Work out the finished part from the listing and answer in its coordinate system (mm). A direction names the side the tool comes from. Coordinates: 2 decimals unless noted, no trailing zeros. Write each loop counter-clockwise with the first axis right and the second up, starting at its lowest first coordinate (ties: lowest second). Pieces come first, ordered by that corner, then holes. Notation, with made-up numbers: M 14.25,-25 L 61.25,-25 A12 cw 61.25,-6 Z; hole C 35,50.25 d2. An arc over 180 degrees is marked long. Use CSV: the item, a comma, the result in double quotes.
from build123d import *

# Parameters (mm, degrees)
F0_R     = 11
F1_DEPTH = 5
F3_DEPTH = 3.5
F5_DEPTH = 14.501
F6_R     = 2.5
F7_DEPTH = 14.501
F8_R     = 8
F9_DEPTH = 25
F10_SIZE = 2


with BuildPart() as f1:
    # F0 (on Top) → F1 (new body)
    with BuildSketch(Plane.XY):
        Circle(F0_R)
    extrude(amount=F1_DEPTH)

    # F2 (on Right) → F3 (join, symmetric)
    with BuildSketch(Plane.YZ):
        Polygon((-11, 5), (0, 5), (11, 5), (11, 40), (-11, 40), align=None)
    extrude(amount=F3_DEPTH, both=True)

    # F4 (on face) → F5 (cut, through all)
    with BuildSketch(Plane.YZ.offset(3.5)):
        Polygon((-11, 35), (0, 40), (-11, 40), align=None)
    extrude(amount=-F5_DEPTH, mode=Mode.SUBTRACT)

    # F6 (on face) → F7 (cut, through all)
    with BuildSketch(Plane.YZ.offset(3.5)):
        with Locations((0, 20)):
            Circle(F6_R)
    extrude(amount=-F7_DEPTH, mode=Mode.SUBTRACT)

    # F8 (on face) → F9 (join)
    with BuildSketch(Plane(origin=(0, 0, 0), x_dir=(1, 0, 0), z_dir=(0, 0, -1))):
        Circle(F8_R)
    extrude(amount=F9_DEPTH)

    # F10
    f10_edges = [f1.edges().sort_by_distance(p)[0] for p in [
        (-8, 0, -25),
    ]]
    chamfer(f10_edges, length=F10_SIZE)


solid = f1.part
Item 1: Consider probe 1 along Z at (x, y) = (1.5, 0); probe 2 along X at (y, z) = (-6.75, 34); probe 3 along Z at (x, y) = (9.5, 5.25). Determine where each line is inside the solid, lowest interval first.
Answer:
probe 1,"z = -25 to 17.5, 22.5 to 40"
probe 2,"x = -3.5 to 3.5"
probe 3,"z = 0 to 5"
Item 2: A tool of negligible diameter and unlimited length cuts with its end or side. For faces 4 (the face through (3.5, 0, 23)), 5 (the face through (-6, 0, 5)), 6 (the face through (-2, -8, 0)), 7 (the face through (0.049, -5.577, 37.465)), from which of +Z, -Z, +X, -X, +Y, -Y can it reach the whole face along a straight path? Write none if from no direction.
Answer:
face 4,"+Z, +X, +Y, -Y"
face 5,"+Z, -X, +Y, -Y"
face 6,"-Z"
face 7,"+Z, +X, -X, -Y"
Item 3: For a pull along Z with two mould halves and no side action, classify faces 1 (the face through (0, 11, 22)), 2 (the face through (0.05, -0.33, 22.48)), 3 (the face through (6, 0, 5)) as released by +Z, released by -Z, zero draft, split by the parting line, or undercut.
Answer:
face 1,"zero draft"
face 2,"undercut"
face 3,"released by +Z"
Item 4: Given pin 1 (8 mm diameter, centred on x = 9, y = 3, fed in from +Z); pin 2 (8 mm diameter, centred on y = -2, z = -8, fed in from +X); pin 3 (12 mm diameter, centred on y = 8.5, z = 31.5, fed in from +X), each flat-ended and moving along its own axis, determine where each tip first touches the part or whether it passes through.
Answer:
pin 1,"stops at z = 5"
pin 2,"stops at x = 8"
pin 3,"stops at x = 3.5"
Item 5: The part is cut by section A-A (z = 21.5). Write down the section's boundary in (x, y).
Answer:
outline,"M -3.5,-11 L 3.5,-11 L 3.5,-2 L -3.5,-2 Z; M -3.5,2 L 3.5,2 L 3.5,11 L -3.5,11 Z"
Item 6: The part is cut by section B-B (z = 10). Write down the section's boundary in (x, y).
Answer:
outline,"M -3.5,-11 L 3.5,-11 L 3.5,11 L -3.5,11 Z"
Item 7: The part is cut by section C-C (y = -9.5). Write down the section's boundary in (x, z).
Answer:
outline,"M -5.55,0 L 5.55,0 L 5.55,5 L 3.5,5 L 3.5,35.68 L -3.5,35.68 L -3.5,5 L -5.55,5 Z"
Item 8: The part is cut by section D-D (x = 8.75). Write down the section's boundary in (y, z), then the cut area to 3 significant figures.
Answer:
outline,"M -6.67,0 L 6.67,0 L 6.67,5 L -6.67,5 Z"
area,"66.7 mm2"
